```python
from build123d import *

# Parameters (mm, degrees)
LINK2OUTERLIP_W     = 50.8
LINK2OUTERLIP_H     = 25.4
LINK2OUTERLIP_W_2   = 44.45
LINK2OUTERLIP_H_2   = 19.05
EXTRUDE_THIN1_DEPTH = 215.9
BOSS_EXTRUDE1_DEPTH = 3.175
BOSS_EXTRUDE2_DEPTH = 3.175
SKETCH4_R           = 3.175
CUT_EXTRUDE1_DEPTH  = 50.8


with BuildPart() as part:
    # Link2OuterLip → Extrude-Thin1 (new body)
    with BuildSketch(Plane.XY):
        Rectangle(LINK2OUTERLIP_W, LINK2OUTERLIP_H)
        Rectangle(LINK2OUTERLIP_W_2, LINK2OUTERLIP_H_2, mode=Mode.SUBTRACT)
    extrude(amount=EXTRUDE_THIN1_DEPTH)

    # Sketch2 → Boss-Extrude1 (add)
    with BuildSketch(Plane.ZY.offset(25.4)):
        with BuildLine():
            Line((0, -12.7), (0, 12.7))
            ThreePointArc((0, 12.7), (-12.7, 0), (0, -12.7))
        make_face()
    boss_extrude1 = extrude(amount=-BOSS_EXTRUDE1_DEPTH)

    # Sketch3 → Boss-Extrude2 (add)
    with BuildSketch(Plane(origin=(25.4, 0, 0), x_dir=(0, 0, -1), z_dir=(1, 0, 0))):
        with BuildLine():
            Line((0, 12.7), (0, -12.7))
            ThreePointArc((0, -12.7), (12.7, 0), (0, 12.7))
        make_face()
    boss_extrude2 = extrude(amount=-BOSS_EXTRUDE2_DEPTH)

    # Sketch4 → Cut-Extrude1 (cut)
    with BuildSketch(Plane(origin=(25.4, 0, 0), x_dir=(0, 0, -1), z_dir=(1, 0, 0))):
        Circle(SKETCH4_R)
    cut_extrude1 = extrude(amount=-CUT_EXTRUDE1_DEPTH, mode=Mode.SUBTRACT)

    # Mirror1: Boss-Extrude1, Boss-Extrude2, Cut-Extrude1 across plane
    add(boss_extrude1.mirror(Plane.XY.offset(107.95)))
    add(boss_extrude2.mirror(Plane.XY.offset(107.95)))
    add(cut_extrude1.mirror(Plane.XY.offset(107.95)), mode=Mode.SUBTRACT)


solid = part.part
```
Work out the finished part from the listing and answer in its coordinate system (mm). A direction names the side the tool comes from. Round coordinates to 2 decimals unless told otherwise and drop trailing zeros. Loops run counter-clockwise (first coordinate to the right, second up) from the corner with the lowest first, then second, coordinate; pieces in that order, holes last. Notation, with made-up numbers: M -12,-16.75 L 10,-16.75 A14 ccw 10,7.25 Z; hole C 45.5,9 d1. An arc over 180 degrees is marked long. Use CSV: the item, a comma, the result in double quotes.
Q1. The mould has two halves that part along Z. Classify faces 1 (the cylindrical face through (23.83, -3.1, 0.69)), 2 (the flat face through (-25.4, 0, 110)), 3 (the cylindrical face through (23.835, -0.279, 228.597)): pulls with the +Z half, pulls with the -Z half, needs draft (parallel to the pull), parting line crosses it, or undercut.
Determined:
face 1,"undercut"
face 2,"needs draft"
face 3,"pulls with the +Z half"
Q2. A tool of negligible diameter and unlimited length cuts with its end or side. For faces 4 (the flat face through (0, 9.525, 106)), 5 (the cylindrical face through (-23.835, 0.279, 228.597)), from which of +Z, -Z, +X, -X, +Y, -Y can it reach the whole face along a straight path? Write none if from no direction.
Determined:
face 4,"+Z, -Z"
face 5,"+Z, +X, -X"
Q3. Section A-A, the plane z = 53 is taken. Determine the outline of the cut face in (x, y) (3 decimals), then the cut area to 3 significant figures.
Determined:
outline,"M -25.4,-12.7 L 25.4,-12.7 L 25.4,12.7 L -25.4,12.7 Z; hole M -22.225,-9.525 L 22.225,-9.525 L 22.225,9.525 L -22.225,9.525 Z"
area,"444 mm2"
Q4. Consider L1, parallel to Y at x = 24.45, z = 0 (3 decimals); L2, parallel to X at y = 5.25, z = 141 (3 decimals); L3, parallel to Y at x = -20, z = 174.5 (3 decimals). Determine where each line is inside the solid, lowest interval first.
Determined:
L1,"-12.7 to -3.175, 3.175 to 12.7"
L2,"-25.4 to -22.225, 22.225 to 25.4"
L3,"-12.7 to -9.525, 9.525 to 12.7"
Q5. Section C-C, the plane x = 13 is taken. Determine the outline of the cut face in (y, z) (3 decimals), then the cut area to 3 significant figures.
Determined:
outline,"M -12.7,0 L -9.525,0 L -9.525,215.9 L -12.7,215.9 Z; M 9.525,0 L 12.7,0 L 12.7,215.9 L 9.525,215.9 Z"
area,"1,370 mm2"
Q6. Each of these flat-tipped pins is pushed along its axis until it touches: pin 1 (1 mm diameter, centred on x = -2, y = -11.5, fed in from -Z); pin 2 (7.5 mm diameter, centred on y = 0, z = 215.9, fed in from -X); pin 3 (1.6 mm diameter, centred on x = -2, y = -11.5, fed in from +Z). Where does it stop, or does it pass through?
Determined:
pin 1,"z = 0"
pin 2,"x = -25.4"
pin 3,"z = 215.9"
Q7. Section B-B, the plane y = 0 is taken. Determine the outline of the cut face in (x, z) (3 decimals).
Determined:
outline,"M -25.4,-12.7 L -22.225,-12.7 L -22.225,-3.175 L -25.4,-3.175 Z; M -25.4,3.175 L -22.225,3.175 L -22.225,212.725 L -25.4,212.725 Z; M -25.4,219.075 L -22.225,219.075 L -22.225,228.6 L -25.4,228.6 Z; M 22.225,-12.7 L 25.4,-12.7 L 25.4,-3.175 L 22.225,-3.175 Z; M 22.225,3.175 L 25.4,3.175 L 25.4,212.725 L 22.225,212.725 Z; M 22.225,219.075 L 25.4,219.075 L 25.4,228.6 L 22.225,228.6 Z"
